Read the model definition and answer for the solid it produces. Units are mm, in the model's axes. Face numbers are marked on the shaded views. A direction names the side the tool comes from. Coordinates: 2 decimals unless noted, no trailing zeros. Loops run counter-clockwise (first coordinate to the right, second up) from the corner with the lowest first, then second, coordinate; pieces in that order, holes last.
Autodesk Inventor part; units mm, degrees
ref_plane "YZ Plane" through (0, 0, 0) normal (1, 0, 0) x (0, 1, 0)
ref_plane "XZ Plane" through (0, 0, 0) normal (0, 1, 0) x (-1, 0, 0)
ref_plane "XY Plane" through (0, 0, 0) normal (0, 0, 1) x (1, 0, 0)
sketch "Sketch1" plane through (0, 0, 0) normal (0, 1, 0) x (-1, 0, 0)
  point P0 (0, 0)
sketch "Sketch2" plane through (0, 0, 0) normal (0, 1, 0) x (-1, 0, 0)
  line L0 (0, 0) -> (85.5, 0)
  line L1 (85.5, 0) -> (85.5, -127.8)
  line L2 (85.5, -127.8) -> (0, -127.8)
  line L3 (0, -127.8) -> (0, 0)
  dimension "d0" = 85.5
  dimension "d1" = 127.8
extrude "Extrusion1" add sketch "Sketch2" along normal blind 15
sketch "Sketch3" plane through (0, 15, 0) normal (0, 1, 0) x (1, 0, 0)
  point P0 (0, 0)
sketch "Sketch5" plane through (0, 15, 0) normal (0, 1, 0) x (1, 0, 0)
  line L0 (0, 127.8) -> (-85.5, 127.8)
  line L1 (-85.5, 127.8) -> (-85.5, 0)
  line L2 (0, 127.8) -> (-85.5, 127.8)
  line L3 (-85.5, 127.8) -> (-85.5, 124.64)
  line L4 (-85.5, 124.64) -> (0, 124.64)
  line L5 (0, 124.64) -> (0, 127.8)
  line L6 (0, 124.64) -> (-85.5, 124.64)
  line L7 (-85.5, 124.64) -> (-85.5, 96.64)
  line L8 (-85.5, 96.64) -> (0, 96.64)
  line L9 (0, 96.64) -> (0, 124.64)
  line L10 (0, 96.64) -> (-85.5, 96.64)
  line L11 (-85.5, 96.64) -> (-85.5, 93.48)
  line L12 (-85.5, 93.48) -> (0, 93.48)
  line L13 (0, 93.48) -> (0, 96.64)
  line L14 (0, 93.48) -> (-85.5, 93.48)
  line L15 (-85.5, 93.48) -> (-85.5, 65.48)
  line L16 (-85.5, 65.48) -> (0, 65.48)
  line L17 (0, 65.48) -> (0, 93.48)
  line L18 (0, 65.48) -> (-85.5, 65.48)
  line L19 (-85.5, 65.48) -> (-85.5, 62.32)
  line L20 (-85.5, 62.32) -> (0, 62.32)
  line L21 (0, 62.32) -> (0, 65.48)
  line L22 (0, 62.32) -> (-85.5, 62.32)
  line L23 (-85.5, 62.32) -> (-85.5, 34.32)
  line L24 (-85.5, 34.32) -> (0, 34.32)
  line L25 (0, 34.32) -> (0, 62.32)
  line L26 (0, 34.32) -> (-85.5, 34.32)
  line L27 (-85.5, 34.32) -> (-85.5, 31.16)
  line L28 (-85.5, 31.16) -> (0, 31.16)
  line L29 (0, 31.16) -> (0, 34.32)
  line L30 (0, 31.16) -> (-85.5, 31.16)
  line L31 (-85.5, 31.16) -> (-85.5, 3.16)
  line L32 (-85.5, 3.16) -> (0, 3.16)
  line L33 (0, 3.16) -> (0, 31.16)
  line L34 (0, 0) -> (0, 127.8)
  line L35 (-85.5, 0) -> (0, 0)
  line L36 (0, 127.8) -> (-0.375, 127.8)
  line L37 (-0.375, 127.8) -> (-0.375, 0)
  line L38 (-0.375, 0) -> (0, 0)
  line L39 (0, 0) -> (0, 127.8)
  line L40 (-0.375, 0) -> (-28.375, 0)
  line L41 (-28.375, 0) -> (-28.375, 127.8)
  line L42 (-28.375, 127.8) -> (-0.375, 127.8)
  line L43 (-0.375, 127.8) -> (-0.375, 0)
  line L44 (-28.375, 127.8) -> (-28.75, 127.8)
  line L45 (-28.75, 127.8) -> (-28.75, 3.16)
  line L46 (-28.75, 3.16) -> (-28.375, 3.16)
  line L47 (-28.375, 3.16) -> (-28.375, 127.8)
  line L48 (-28.75, 127.8) -> (-56.75, 127.8)
  line L49 (-56.75, 127.8) -> (-56.75, 3.16)
  line L50 (-56.75, 3.16) -> (-28.75, 3.16)
  line L51 (-28.75, 3.16) -> (-28.75, 127.8)
  line L52 (-56.75, 127.8) -> (-57.125, 127.8)
  line L53 (-57.125, 127.8) -> (-57.125, 3.16)
  line L54 (-57.125, 3.16) -> (-56.75, 3.16)
  line L55 (-56.75, 3.16) -> (-56.75, 127.8)
  line L56 (-57.125, 127.8) -> (-85.125, 127.8)
  line L57 (-85.125, 127.8) -> (-85.125, 3.16)
  line L58 (-85.125, 3.16) -> (-57.125, 3.16)
  line L59 (-57.125, 3.16) -> (-57.125, 127.8)
  circle A0 centre (-14.375, 110.64) radius 14
  circle A1 centre (-14.375, 79.48) radius 14
  circle A2 centre (-14.375, 48.32) radius 14
  circle A3 centre (-14.375, 17.16) radius 14
  circle A4 centre (-42.75, 110.64) radius 14
  circle A5 centre (-42.75, 79.48) radius 14
  circle A6 centre (-42.75, 48.32) radius 14
  circle A7 centre (-42.75, 17.16) radius 14
  circle A8 centre (-71.125, 17.16) radius 14
  circle A9 centre (-71.125, 48.32) radius 14
  circle A10 centre (-71.125, 79.48) radius 14
  circle A11 centre (-71.125, 110.64) radius 14
  dimension "d22" = 3.16
  dimension "d23" = 28
  dimension "d24" = 3.16
  dimension "d25" = 28
  dimension "d26" = 3.16
  dimension "d27" = 28
  dimension "d28" = 3.16
  dimension "d29" = 28
  dimension "d30" = 0.375
  dimension "d31" = 28
  dimension "d32" = 0.375
  dimension "d33" = 28
  dimension "d34" = 0.375
  dimension "d35" = 28
extrude "Extrusion3" cut sketch "Sketch5" against normal blind 10 contours A0 | A4 | A1 | A11 | A2 | A5 | A3 | A10 | A6 | A7 | A9 | A8
properties part number "scintillationvialholder2"
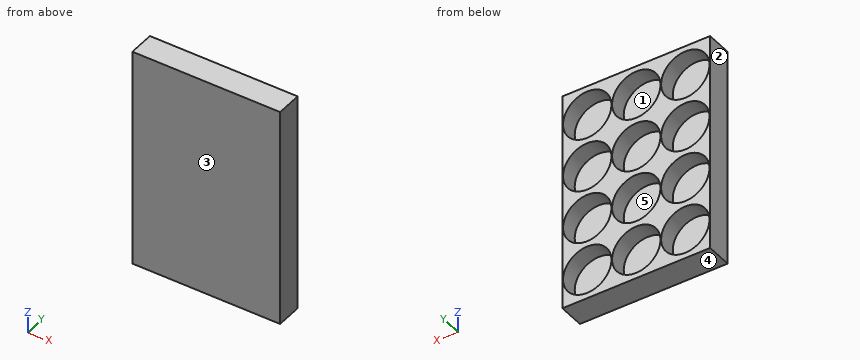
Q1. A cutting plane is placed at D-D (z = -86). Give the vertices of the cut face in (x, y).
Findings below:
outline: (-85.5, 0) - (0, 0) - (0, 15) - (-1.99, 15) - (-1.99, 5) - (-26.76, 5) - (-26.76, 15) - (-30.36, 15) - (-30.36, 5) - (-55.14, 5) - (-55.14, 15) - (-58.74, 15) - (-58.74, 5) - (-83.51, 5) - (-83.51, 15) - (-85.5, 15) - close
Q2. A flat-ended cylindrical pin translates along its axis: pin 1 Ø8 at (x, z) = (-34, -14.5) entering from +Y. Find the tip coordinate at first contact, or state that the pin passes through.
Findings below:
pin 1: stops at y = 5
Q3. Straight lines are drawn through the part: probe 1 along X at (y, z) = (12.25, -79.48) (3 decimals); probe 2 along Z at (x, y) = (-42.75, 12); probe 3 along X at (y, z) = (13.75, -29). For each, find the intervals that lie inside material, in ascending order.
Findings below:
probe 1: x = -85.5 to -85.125, -57.125 to -56.75, -28.75 to -28.375, -0.375 to 0
probe 2: z = -127.8 to -124.64, -96.64 to -93.48, -65.48 to -62.32, -34.32 to -31.16, -3.16 to 0
probe 3: x = -85.5 to -78.6, -63.65 to -50.22, -35.28 to -21.85, -6.9 to 0
Q4. Determine the mould class of the marked faces 1, 2 and 3 for opening direction X: +X half, -X half, draft (parallel to the pull), parting line (faces both ways), or undercut.
Findings below:
face 1: undercut
face 2: -X half
face 3: draft
Q5. A cutting plane is placed at B-B (y = 10.75). Count the separate pieces of the cut face and the enclosed holes in it, then the cut area to 3 significant figures.
Findings below:
separate pieces: 1
enclosed holes: 12
area: 3,540 mm2
Q6. Which of the six approach directions +Z, -Z, +X, -X, +Y, -Y give full straight-line access (tool end or side, diameter ignored) to the marked faces 4 and 5?
Findings below:
face 4: -Z, +X, -X, +Y, -Y
face 5: +Y
Q7. A cutting plane is placed at C-C (x = -42.75). Give the vertices of the cut face in (y, z).
Findings below:
outline: (0, -127.8) - (15, -127.8) - (15, -124.64) - (5, -124.64) - (5, -96.64) - (15, -96.64) - (15, -93.48) - (5, -93.48) - (5, -65.48) - (15, -65.48) - (15, -62.32) - (5, -62.32) - (5, -34.32) - (15, -34.32) - (15, -31.16) - (5, -31.16) - (5, -3.16) - (15, -3.16) - (15, 0) - (0, 0) - close
Q8. A cutting plane is placed at A-A (z = -17.16). Give the vertices of the cut face in (x, y) (3 decimals), then the cut area to 4 significant figures.
Findings below:
outline: (-85.5, 0) - (0, 0) - (0, 15) - (-0.375, 15) - (-0.375, 5) - (-28.375, 5) - (-28.375, 15) - (-28.75, 15) - (-28.75, 5) - (-56.75, 5) - (-56.75, 15) - (-57.125, 15) - (-57.125, 5) - (-85.125, 5) - (-85.125, 15) - (-85.5, 15) - close
area: 442.5 mm2
